```python
from build123d import *

# Parameters (mm, degrees)
BOSS_EXTRUDE1_DEPTH = 2.5
SKETCH2_R           = 1
CUT_EXTRUDE1_DEPTH  = 4.5
SKETCH3_R           = 1
CUT_EXTRUDE2_DEPTH  = 9.5
SKETCH5_R           = 1
BOSS_EXTRUDE2_DEPTH = 9.5


with BuildPart() as part:
    # Sketch1 → Boss-Extrude1 (new body)
    with BuildSketch(Plane.XY):
        Polygon((-70.406172668, -77.710060133), (-55.350496572, -77.710060133), (-55.155758053, -77.477979804), (-53.240646945, -79.084948828), (-54.184487309, -80.209773972), (-70.368347793, -80.209773972), align=None)
    extrude(amount=BOSS_EXTRUDE1_DEPTH)

    # Sketch2 → Cut-Extrude1 (cut)
    with BuildSketch(Plane(origin=(-60.939488189, -72.62485398, 0), x_dir=(0, 0, -1), z_dir=(0.6427876096865354, 0.7660444431189815, 0))):
        with Locations(Location((-1.25, -8.800123479, 0), (0, 0, 90))):
            Circle(SKETCH2_R)
    extrude(amount=-CUT_EXTRUDE1_DEPTH, mode=Mode.SUBTRACT)

    # Sketch3 → Cut-Extrude2 (cut)
    with BuildSketch(Plane(origin=(-71.565670343, -1.082908957, 0), x_dir=(0, 0, 1), z_dir=(-0.9998855357578961, -0.015129949839474953, 0))):
        with Locations(Location((1.25, -77.885923249, 0), (0, 0, 270))):
            Circle(SKETCH3_R)
    extrude(amount=-CUT_EXTRUDE2_DEPTH, mode=Mode.SUBTRACT)

    # Sketch5 → Boss-Extrude2 (add)
    with BuildSketch(Plane(origin=(-71.565670343, -1.082908957, 0), x_dir=(0, 0, 1), z_dir=(-0.9998855357578961, -0.015129949839476386, 0))):
        with Locations((1.25, -77.885923249)):
            Circle(SKETCH5_R)
    extrude(amount=-BOSS_EXTRUDE2_DEPTH)


solid = part.part
```
Verification items for the finished model (mm, model axes). Coordinates: 2 decimals unless noted, no trailing zeros. Write each loop counter-clockwise with the first axis right and the second up, starting at its lowest first coordinate (ties: lowest second). Pieces come first, ordered by that corner, then holes. Notation, with made-up numbers: M 62,78 L 83,78 A14 ccw 83,88 Z; hole C 43.25,70.25 d7. An arc over 180 degrees is marked long. Answer as a JSON object with one key per item and string values. Group by question number.
(1) Gauge pin test, flat end, axial feed: pin 1 (1.2 mm diameter, centred on x = -65.5, z = 1.5, fed in from +Y). Record the tip position at first contact, or that the pin passes through.
(2) Release check for a two-part mould opening along X. For faces 1 (the face through (-53.706, -79.639, 1.232)), 2 (the face through (-55.75, -78.65, 1.55)), 3 (the face through (-63, -77.71, 1)) record: +X half, -X half, draft (parallel to the pull), parting line (faces both ways), or undercut.
(3) Cross-section at A-A, the plane z = 1.6. Record the cut outline in (x, y), and give its area (3 significant figures).
(4) Cross-section at B-B, the plane x = -60. Record the cut outline in (y, z).
(5) Material ranges on line 1 (X direction, y = -80.05, z = 1); line 2 (Y direction, x = -62.5, z = 2.15); line 3 (X direction, y = -78.95, z = 1.7), recorded low to high.
Reply:
{
 "1": {"pin 1": "y = -77.71"},
 "2": {"face 1": "+X half", "face 2": "undercut", "face 3": "draft"},
 "3": {"outline": "M -70.41,-77.71 L -70.37,-80.21 L -57.04,-80.21 L -54.92,-77.68 L -55.16,-77.48 L -55.35,-77.71 Z; M -54.59,-80.21 L -54.18,-80.21 L -53.24,-79.08 L -53.48,-78.88 Z", "area": "36.5 mm²"},
 "4": {"outline": "M -80.21,0 L -77.71,0 L -77.71,2.5 L -80.21,2.5 Z"},
 "5": {"line 1": "-70.37 to -56.95, -54.42 to -54.05", "line 2": "-80.21 to -77.71", "line 3": "-70.39 to -55.92, -53.59 to -53.4"}
}
